Input: part model. Units: mm. Frame: model coordinates. Give positions to 0.01 mm unless a question says otherwise; leave off trailing zeros. Write each loop counter-clockwise with the first axis right and the second up, starting at its lowest first coordinate (ties: lowest second). Pieces come first, ordered by that corner, then holes. Notation, with made-up numbers: (15, 13.5) -> (21, 13.5) arc R23 ccw to (21, 51.5) -> close; hole circle Ø5 at (27.5, 41). An arc over 180 degrees is marked (long way). Return JSON: item names as keys, results as strings. Group by question number.
Item 1: Section C-C, the plane y = 5.5. Return loops of the section in (x, z).
Item 2: Pin query (flat end, axial travel): P1, Ø12, axis at x = -94.5, y = -46, coming from the +Z side; P2, Ø1, axis at y = -61, z = 2, coming from the -X side. Return the tip coordinate at first contact, or that it passes through.
Item 3: Line query: line 1 (Z direction, x = -143.5, y = 68.5). Output: solid intervals per line, ascending. Write a range as [from, to].
Item 4: Section B-B, the plane x = -16.5. Return loops of the section in (y, z).
Item 5: Section A-A, the plane z = 2.35. Return loops of the section in (x, y).
from build123d import *

# Parameters (mm, degrees)
PAD_DEPTH    = 1
SKETCH001_R  = 1.35
PAD001_DEPTH = 6
SKETCH003_R  = 1.35
PAD002_DEPTH = 6
SKETCH002_R  = 1.35
PAD003_DEPTH = 6
SKETCH004_R  = 1.35
PAD004_DEPTH = 6


with BuildPart() as part:
    # Sketch → Pad (new body)
    with BuildSketch(Plane.XY):
        with BuildLine():
            Line((-181.5, 76.5), (-181.5, -76.5))
            ThreePointArc((-181.5, -76.5), (-180.035534, -80.035534), (-176.5, -81.5))
            Line((-176.5, -81.5), (176.5, -81.5))
            ThreePointArc((176.5, -81.5), (180.035534, -80.035534), (181.5, -76.5))
            Line((181.5, -76.5), (181.5, 76.5))
            ThreePointArc((181.5, 76.5), (180.035534, 80.035534), (176.5, 81.5))
            Line((176.5, 81.5), (-176.5, 81.5))
            ThreePointArc((-176.5, 81.5), (-180.035534, 80.035534), (-181.5, 76.5))
        make_face()
    extrude(amount=PAD_DEPTH)

    # Sketch001 → Pad001 (join)
    with BuildSketch(Plane.XY):
        with Locations((-175, 75)):
            Circle(SKETCH001_R)
    extrude(amount=PAD001_DEPTH)

    # Sketch003 → Pad002 (join)
    with BuildSketch(Plane.XY):
        with Locations((175, 75)):
            Circle(SKETCH003_R)
    extrude(amount=PAD002_DEPTH)

    # Sketch002 → Pad003 (join)
    with BuildSketch(Plane.XY):
        with Locations((-175, -75)):
            Circle(SKETCH002_R)
    extrude(amount=PAD003_DEPTH)

    # Sketch004 → Pad004 (join)
    with BuildSketch(Plane.XY):
        with Locations((175, -75)):
            Circle(SKETCH004_R)
    extrude(amount=PAD004_DEPTH)


solid = part.part
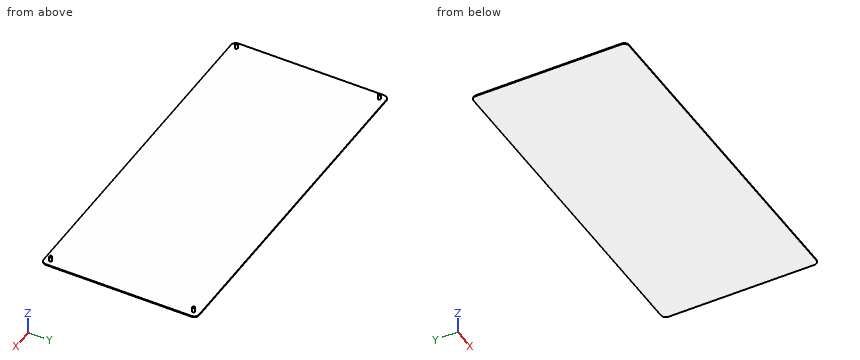
Answer below:
{
 "1": {"outline": "(-181.5, 0) -> (181.5, 0) -> (181.5, 1) -> (-181.5, 1) -> close"},
 "2": {"P1": "stops at z = 1", "P2": "passes through"},
 "3": {"line 1": "z = [0, 1]"},
 "4": {"outline": "(-81.5, 0) -> (81.5, 0) -> (81.5, 1) -> (-81.5, 1) -> close"},
 "5": {"outline": "circle Ø2.7 at (-175, -75); circle Ø2.7 at (-175, 75); circle Ø2.7 at (175, -75); circle Ø2.7 at (175, 75)"}
}
